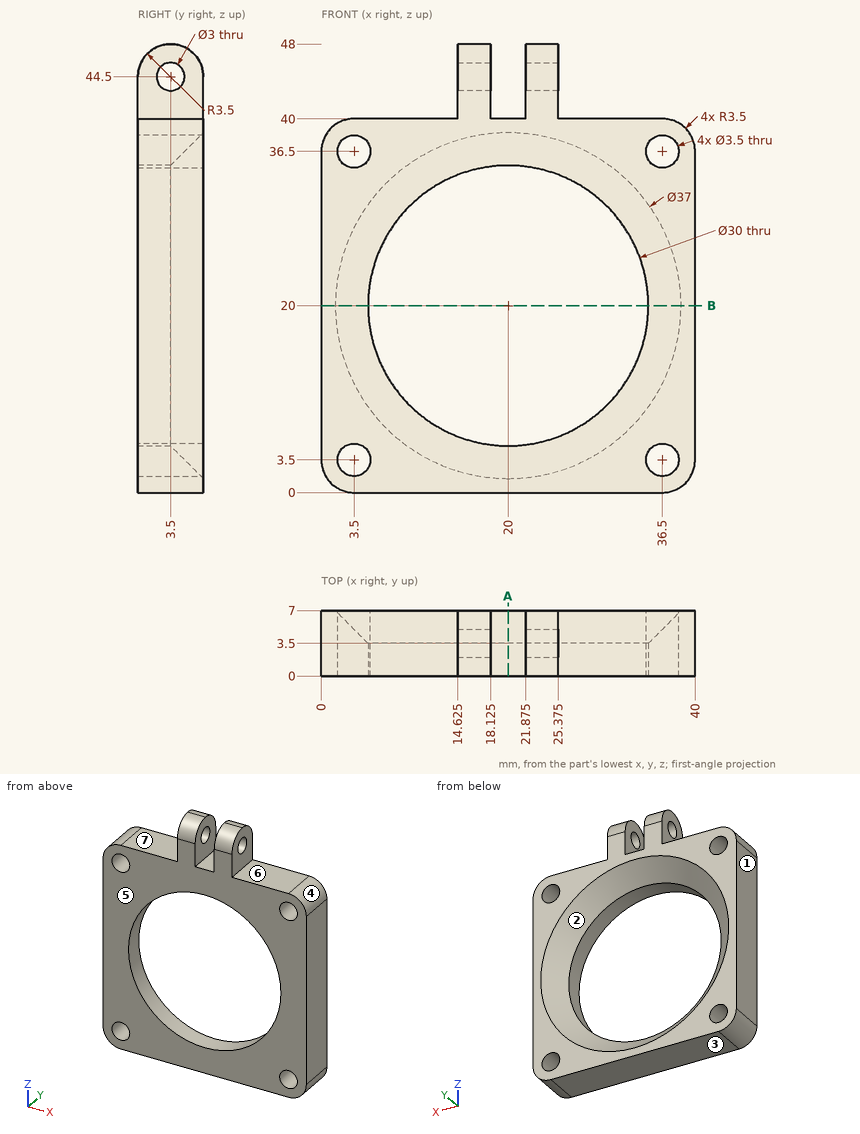
Geometry: see drawing. Coordinates: mm, zero at the bounding-box minimum. A direction names the side the tool comes from. Coordinates: 2 decimals unless noted, no trailing zeros. Loops run counter-clockwise (first coordinate to the right, second up) from the corner with the lowest first, then second, coordinate; pieces in that order, holes last. Notation, with made-up numbers: (-14.75, 85.5) - (4.25, 85.5) arc R21 ccw to (4.25, 109.5) - close; hole circle Ø9 at (61.25, 67.25). An arc over 180 degrees is marked (long way). Answer as CSV lines item,"result".
1. Section B-B (z = 20). Return loops of the section in (x, y).
Established:
outline,"(0, 0) - (5, 0) - (5, 3.5) - (1.5, 7) - (0, 7) - close; (35, 0) - (40, 0) - (40, 7) - (38.5, 7) - (35, 3.5) - close"
2. Mould query, pull axis Z, two halves, no side actions, for the marked faces 1, 2, 3 and 4. Classes: released by +Z, released by -Z, zero draft, split by the parting line, or undercut.
Established:
face 1,"zero draft"
face 2,"undercut"
face 3,"released by -Z"
face 4,"released by +Z"
3. Ray query, line 1 (X direction, y = 3, z = 36.5); line 2 (X direction, y = 1.5, z = 43) (3 decimals); line 3 (Z direction, x = 2, y = 5.75). Return the intervals inside material, ascending.
Established:
line 1,"x = 0 to 1.75, 5.25 to 34.75, 38.25 to 40"
line 2,"x = 14.625 to 18.125, 21.875 to 25.375"
line 3,"z = 0.34 to 2.6, 4.4 to 35.6, 37.4 to 39.66"
4. Contact query for flat-ended pins moving along their axis: pin 1 (1.1 mm diameter, centred on x = 20, y = 2, fed in from +Z); pin 2 (4 mm diameter, centred on x = 27, y = 1, fed in from -Z); pin 3 (3.5 mm diameter, centred on y = 3, z = 45, fed in from -X) (3 decimals); pin 4 (4 mm diameter, centred on y = 3.5, z = 44.5, fed in from +X) (3 decimals). Output: stop coordinate, or through.
Established:
pin 1,"stops at z = 40"
pin 2,"stops at z = 0"
pin 3,"stops at x = 14.625"
pin 4,"stops at x = 25.375"
5. Reachability of the marked faces 5, 6 and 7 from +Z, -Z, +X, -X, +Y, -Y: full face, straight path, thin tool, end or side. Return the list, or none.
Established:
face 5,"+Z, -Z, +X, -X, -Y"
face 6,"+Z, +X, +Y, -Y"
face 7,"+Z, -X, +Y, -Y"
6. Section A-A (x = 20). Return loops of the section in (y, z).
Established:
outline,"(0, 0) - (7, 0) - (7, 1.5) - (3.5, 5) - (0, 5) - close; (0, 35) - (3.5, 35) - (7, 38.5) - (7, 40) - (0, 40) - close"
